Source: three-view drawing plus pictorial views. Frame: mm from the lowest corner of the part. A direction names the side the tool comes from. Coordinates: 2 decimals unless noted, no trailing zeros. Loops run counter-clockwise (first coordinate to the right, second up) from the corner with the lowest first, then second, coordinate; pieces in that order, holes last. Notation, with made-up numbers: (-15, 66) - (27, 66) arc R36 ccw to (27, 103) - close; hole circle Ø11 at (-4, 20.25). An arc over 180 degrees is marked (long way). Return JSON: item names as keys, results as strings.
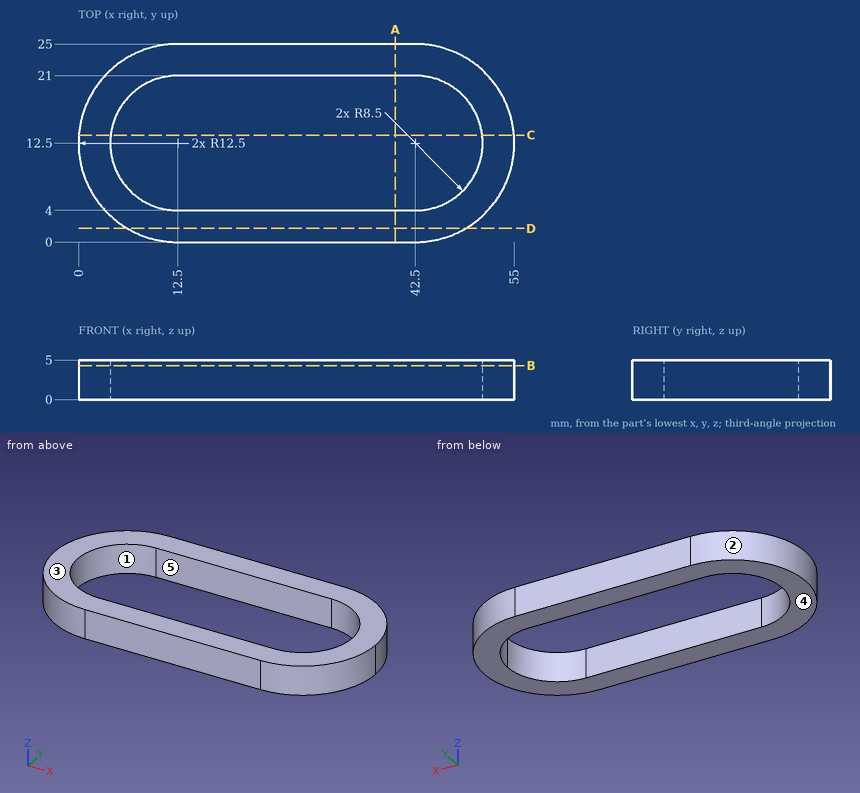
Item 1: Section query B-B, the plane z = 4.3. Return loops of the section in (x, y), and give its area (3 significant figures).
Worked out:
{"outline": "(12.5, 0) - (42.5, 0) arc R12.5 ccw to (55, 12.5) arc R12.5 ccw to (42.5, 25) - (12.5, 25) arc R12.5 ccw to start; hole (12.5, 4) - (42.5, 4) arc R8.5 ccw to (51, 12.5) arc R8.5 ccw to (42.5, 21) - (12.5, 21) arc R8.5 ccw to start", "area": "504 mm^2"}
Item 2: Mould query, pull axis X, two halves, no side actions, for the marked faces 1, 2 and 3. Classes: +X half, -X half, draft (parallel to the pull), parting line (faces both ways), or undercut.
Worked out:
{"face 1": "undercut", "face 2": "-X half", "face 3": "draft"}
Item 3: Reachability of the marked faces 4 and 5 from +Z, -Z, +X, -X, +Y, -Y: full face, straight path, thin tool, end or side. Return the list, or none.
Worked out:
{"face 4": "-Z, +X, -X, +Y, -Y", "face 5": "+Z, -Z"}
Item 4: Ray query, probe 1 along Y at (x, z) = (26, 4.25); probe 2 along X at (y, z) = (20.25, 4.5); probe 3 along X at (y, z) = (14, 4.75). Return the intervals inside material, ascending. Write a range as from..to.
Worked out:
{"probe 1": "0..4, 21..25", "probe 2": "2.69..9.01, 45.99..52.31", "probe 3": "0.09..4.13, 50.87..54.91"}
Item 5: Section query D-D, the plane y = 1.75. Return loops of the section in (x, z), and give its area (3 significant figures).
Worked out:
{"outline": "(6.12, 0) - (48.88, 0) - (48.88, 5) - (6.12, 5) - close", "area": "214 mm^2"}
Item 6: Section query C-C, the plane y = 13.5. Return loops of the section in (x, z).
Worked out:
{"outline": "(0.04, 0) - (4.06, 0) - (4.06, 5) - (0.04, 5) - close; (50.94, 0) - (54.96, 0) - (54.96, 5) - (50.94, 5) - close"}
Item 7: Section query A-A, the plane x = 40. Return loops of the section in (y, z), and give its area (3 significant figures).
Worked out:
{"outline": "(0, 0) - (4, 0) - (4, 5) - (0, 5) - close; (21, 0) - (25, 0) - (25, 5) - (21, 5) - close", "area": "40.0 mm^2"}
